Here's the drawing with two shaded views (mm, measured from the low corner). I have some questions. Give positions to 0.01 mm unless a question says otherwise; leave off trailing zeros. Write each loop counter-clockwise with the first axis right and the second up, starting at its lowest first coordinate (ties: lowest second). Pieces come first, ordered by that corner, then holes.
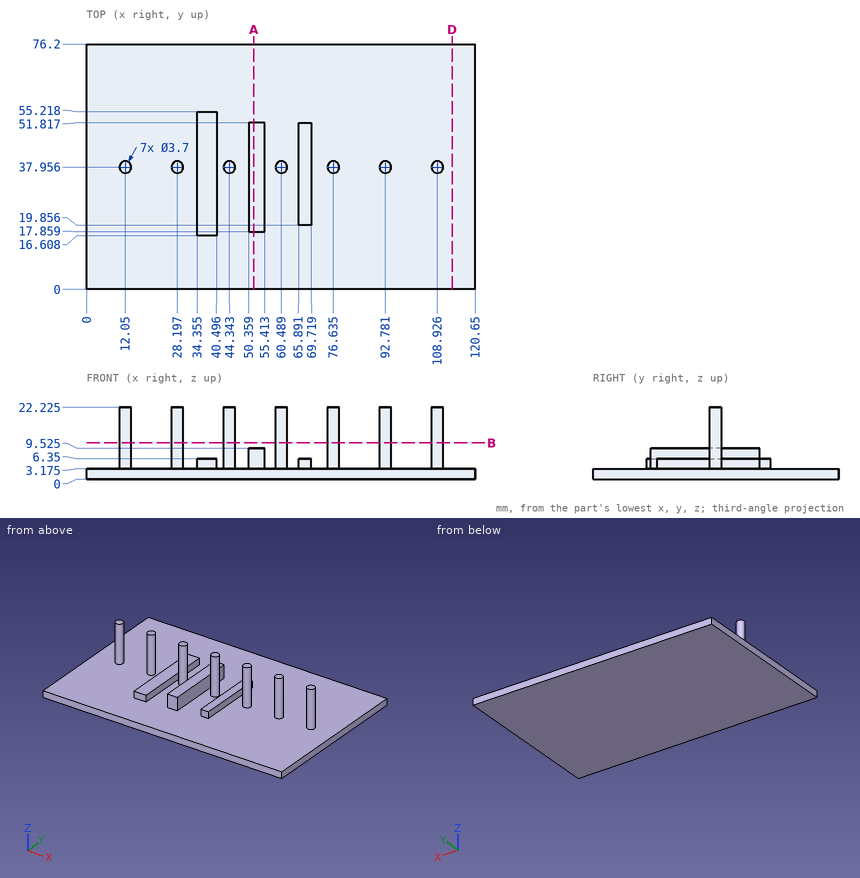
1) Please list where these lines run through material, in increasing order: L1, parallel to X at y = 26, z = 3.75 (1 decimal); L2, parallel to Z at x = 66.5, y = 21.5; L3, parallel to Z at x = 67, y = 60 (1 decimal).
Values follow:
L1: x = 34.4 to 40.5, 50.4 to 55.4, 65.9 to 69.7
L2: z = 0 to 6.35
L3: z = 0 to 3.2
2) For pin 1 Ø5.5 at (x, y) = (53.5, 28.5) entering from +Z (1 decimal); pin 2 Ø1.9 at (y, z) = (38, 5) entering from +X; pin 3 Ø3.5 at (x, z) = (67.5, 4.5) entering from -Y; pin 4 Ø1.6 at (x, z) = (68.5, 5) entering from +Y, each with a flat end and sliding along its axis, tell me the tip position at first contact or that it passes through.
Values follow:
pin 1: stops at z = 9.5
pin 2: stops at x = 110.78
pin 3: stops at y = 0
pin 4: stops at y = 51.82
3) Suppose I cut it at A-A on x = 52. Write out the boundary of the cut face in (y, z) (1 decimal).
Values follow:
outline: (0, 0) - (76.2, 0) - (76.2, 3.2) - (51.8, 3.2) - (51.8, 9.5) - (17.9, 9.5) - (17.9, 3.2) - (0, 3.2) - close
4) Suppose I cut it at B-B on z = 11.25. State how many separate pieces and enclosed holes the cut face has.
Values follow:
separate pieces: 7
enclosed holes: 0
5) Suppose I cut it at D-D on x = 113.5. Write out the boundary of the cut face in (y, z) (1 decimal).
Values follow:
outline: (0, 0) - (76.2, 0) - (76.2, 3.2) - (0, 3.2) - close
